Could you check a few things on this model? Use its own coordinates, in mm. A direction names the side the tool comes from. Round coordinates to 2 decimals unless told otherwise and drop trailing zeros. Write each loop counter-clockwise with the first axis right and the second up, starting at its lowest first coordinate (ties: lowest second). Pieces come first, ordered by that corner, then holes. Notation, with made-up numbers: (85.5, 34) -> (121.5, 34) arc R26 ccw to (121.5, 73) -> close; hole circle Ø5 at (32.25, 43.25). An arc over 180 degrees is marked (long way). Answer in a Markdown table with one row per item.
from build123d import *

# Parameters (mm, degrees)
SKETCH1_R                                    = 2.55
BOSS_EXTRUDE1_DEPTH                          = 10
SKETCH2_R                                    = 5.55
SKETCH2_R_2                                  = 2.55
BOSS_EXTRUDE2_DEPTH                          = 7.6
ENL_V_MAT_EXTRU_1_DEPTH                      = 8
RAINURE_DE_CHAMBRAGE_POUR_VIS_T_TE_RON_DEPTH = 10
RAINURE_DE_CHAMBRAGE_POUR_VIS_T_TE_3_DEPTH   = 3


# Read off the part's stored shape, not the designer's step: Rainure de chambrage pour vis à tête ronde bombée M32
with BuildPart() as part:
    # Sketch1 → Boss-Extrude1 (new body)
    with BuildSketch(Plane.XY):
        with BuildLine():
            Line((14.75, -33.5), (-14.75, -33.5))
            ThreePointArc((-14.75, -33.5), (-18.285533906, -32.035533906), (-19.75, -28.5))
            Line((-19.75, -28.5), (-19.75, 28.5))
            ThreePointArc((-19.75, 28.5), (-18.285533906, 32.035533906), (-14.75, 33.5))
            Line((-14.75, 33.5), (14.75, 33.5))
            ThreePointArc((14.75, 33.5), (18.285533906, 32.035533906), (19.75, 28.5))
            Line((19.75, 28.5), (19.75, -28.5))
            ThreePointArc((19.75, -28.5), (18.285533906, -32.035533906), (14.75, -33.5))
        make_face()
        with Locations((0, 26.5)):
            Circle(SKETCH1_R, mode=Mode.SUBTRACT)
    extrude(amount=BOSS_EXTRUDE1_DEPTH)

    # Sketch2 → Boss-Extrude2 (add)
    with BuildSketch(Plane.XY.offset(10)):
        with Locations(Location((0, 26.5, 0), (0, 0, 180))):
            Circle(SKETCH2_R)
        with Locations((0, 26.5)):
            Circle(SKETCH2_R_2, mode=Mode.SUBTRACT)
    extrude(amount=BOSS_EXTRUDE2_DEPTH)

    # Esquisse1 → Enlèv. mat.-Extru.1 (cut)
    with BuildSketch(Plane(origin=(0, 0, 0), x_dir=(-1, 0, 0), z_dir=(0, 0, -1))):
        Polygon((2.453738644, 22.25), (4.907477288, 26.5), (2.453738644, 30.75), (-2.453738644, 30.75), (-4.907477288, 26.5), (-2.453738644, 22.25), align=None)
    extrude(amount=-ENL_V_MAT_EXTRU_1_DEPTH, mode=Mode.SUBTRACT)

    # Rainure de chambrage pour vis _ t_te 2 → Rainure de chambrage pour vis à tête ronde bombée M32 (cut)
    with BuildSketch(Plane.XY):
        with BuildLine():
            ThreePointArc((1.7, -21.99), (0, -20.29), (-1.7, -21.99))
            Line((-1.7, -21.99), (-1.7, -28.59))
            ThreePointArc((-1.7, -28.59), (0, -30.29), (1.7, -28.59))
            Line((1.7, -28.59), (1.7, -21.99))
        make_face()
        with BuildLine():
            Line((1.7, -8.59), (1.7, -1.99))
            ThreePointArc((1.7, -1.99), (0, -0.29), (-1.7, -1.99))
            Line((-1.7, -1.99), (-1.7, -8.59))
            ThreePointArc((-1.7, -8.59), (0, -10.29), (1.7, -8.59))
        make_face()
    extrude(amount=RAINURE_DE_CHAMBRAGE_POUR_VIS_T_TE_RON_DEPTH, mode=Mode.SUBTRACT)

    # Rainure de chambrage pour vis _ t_te 3 o → Rainure de chambrage pour vis _ t_te 3 (cut)
    # profile 1 of 2: a face of its own
    with BuildSketch(Plane.XY):
        with BuildLine():
            ThreePointArc((3.5, -21.99), (0, -18.49), (-3.5, -21.99))
            Line((-3.5, -21.99), (-3.5, -28.59))
            ThreePointArc((-3.5, -28.59), (0, -32.09), (3.5, -28.59))
            Line((3.5, -28.59), (3.5, -21.99))
        make_face()
        with BuildLine():
            Line((-1.7, -28.59), (-1.7, -21.99))
            ThreePointArc((-1.7, -21.99), (0, -20.29), (1.7, -21.99))
            Line((1.7, -21.99), (1.7, -28.59))
            ThreePointArc((1.7, -28.59), (0, -30.29), (-1.7, -28.59))
        make_face(mode=Mode.SUBTRACT)
    # profile 2 of 2: a face of its own
    with BuildSketch(Plane.XY):
        with BuildLine():
            Line((3.5, -8.59), (3.5, -1.99))
            ThreePointArc((3.5, -1.99), (0, 1.51), (-3.5, -1.99))
            Line((-3.5, -1.99), (-3.5, -8.59))
            ThreePointArc((-3.5, -8.59), (0, -12.09), (3.5, -8.59))
        make_face()
        with BuildLine():
            ThreePointArc((-1.7, -1.99), (0, -0.29), (1.7, -1.99))
            Line((1.7, -1.99), (1.7, -8.59))
            ThreePointArc((1.7, -8.59), (0, -10.29), (-1.7, -8.59))
            Line((-1.7, -8.59), (-1.7, -1.99))
        make_face(mode=Mode.SUBTRACT)
    extrude(amount=RAINURE_DE_CHAMBRAGE_POUR_VIS_T_TE_3_DEPTH, mode=Mode.SUBTRACT)


solid = part.part
1) Thinking about a two-plate mould opening in X: for faces 1 (the face through (1.7, -5, 6)), 2 (the face through (18.32, -32, 4.93)), 3 (the face through (-2.4, 25.2, 17.6)), which applies, +X half, -X half, draft (parallel to the pull), parting line (faces both ways), or undercut?
Findings:
| item | result |
|---|---|
| face 1 | undercut |
| face 2 | +X half |
| face 3 | draft |
2) Please list where these lines run through material, in increasing order: line 1 (X direction, y = 26.5, z = 15); line 2 (Y direction, x = 0, z = 14.25); line 3 (Z direction, x = 11.5, y = 16).
Findings:
| item | result |
|---|---|
| line 1 | x = -5.55 to -2.55, 2.55 to 5.55 |
| line 2 | y = 20.95 to 23.95, 29.05 to 32.05 |
| line 3 | z = 0 to 10 |
3) For pin 1 (2.5 mm diameter, centred on x = -1, y = 26, fed in from -Z); pin 2 (10 mm diameter, centred on x = 2, y = -6, fed in from +Z); pin 3 (6.5 mm diameter, centred on x = 0, y = 26.5, fed in from -Z), each with a flat end and sliding along its axis, tell me the tip position at first contact or that it passes through.
Findings:
| item | result |
|---|---|
| pin 1 | passes through |
| pin 2 | stops at z = 10 |
| pin 3 | stops at z = 8 |
4) Imagine slicing it at A-A, the plane z = 4.25. Please give me the cut outline in (x, y).
Findings:
| item | result |
|---|---|
| outline | (-19.75, -28.5) arc R5 ccw to (-14.75, -33.5) -> (14.75, -33.5) arc R5 ccw to (19.75, -28.5) -> (19.75, 28.5) arc R5 ccw to (14.75, 33.5) -> (-14.75, 33.5) arc R5 ccw to (-19.75, 28.5) -> close; hole (-4.91, 26.5) -> (-2.45, 22.25) -> (2.45, 22.25) -> (4.91, 26.5) -> (2.45, 30.75) -> (-2.45, 30.75) -> close; hole (-1.7, -28.59) arc R1.7 ccw to (1.7, -28.59) -> (1.7, -21.99) arc R1.7 ccw to (-1.7, -21.99) -> close; hole (-1.7, -8.59) arc R1.7 ccw to (1.7, -8.59) -> (1.7, -1.99) arc R1.7 ccw to (-1.7, -1.99) -> close |
5) Imagine slicing it at B-B, the plane x = 0. Count the separate pieces of the cut face and the enclosed holes in it, plus the area to 3 significant figures.
Findings:
| item | result |
|---|---|
| separate pieces | 4 |
| enclosed holes | 0 |
| area | 416 mm^2 |
6) Imagine slicing it at D-D, the plane x = -9. Please give me the cut outline in (y, z), plus the area to 3 significant figures.
Findings:
| item | result |
|---|---|
| outline | (-33.5, 0) -> (33.5, 0) -> (33.5, 10) -> (-33.5, 10) -> close |
| area | 670 mm^2 |
7) Imagine slicing it at C-C, the plane y = -9.5. Please give me the cut outline in (x, z), plus the area to 3 significant figures.
Findings:
| item | result |
|---|---|
| outline | (-19.75, 0) -> (-3.38, 0) -> (-3.38, 3) -> (-1.44, 3) -> (-1.44, 10) -> (-19.75, 10) -> close; (1.44, 3) -> (3.38, 3) -> (3.38, 0) -> (19.75, 0) -> (19.75, 10) -> (1.44, 10) -> close |
| area | 355 mm^2 |
8) For faces 4 (the face through (0, 33.5, 5)), 5 (the face through (-0.04, -30.29, 6.45)), 6 (the face through (-3.663, 24.345, 3.944)), which set-ups out of +Z, -Z, +X, -X, +Y, -Y let a thin tool reach every point of the face, with its end or its side?
Findings:
| item | result |
|---|---|
| face 4 | +Z, -Z, +X, -X, +Y |
| face 5 | +Z, -Z |
| face 6 | -Z |
